from build123d import *

# Parameters (mm, degrees)
F0_R     = 1.6
F0_W     = 60
F0_H     = 15
F1_DEPTH = 2
F2_R     = 3
F3_SIZE  = 0.2


with BuildPart() as f1:
    # F0 (on Front) → F1 (new body)
    with BuildSketch(Plane.XZ):
        Polygon((-45, -57.5), (25, -57.5), (25, 0), (45, 0), (45, 57.5), (-45, 57.5), align=None)
        with Locations((-37.5, -52.5)):
            Circle(F0_R, mode=Mode.SUBTRACT)
        with Locations((-7.5, -52.5)):
            Circle(F0_R, mode=Mode.SUBTRACT)
        with Locations((-4.111738, 18.929576)):
            Rectangle(F0_W, F0_H, mode=Mode.SUBTRACT)
        with Locations((-37.5, 52.5)):
            Circle(F0_R, mode=Mode.SUBTRACT)
        with Locations((37.5, 7.5)):
            Circle(F0_R, mode=Mode.SUBTRACT)
        with Locations((37.5, 52.5)):
            Circle(F0_R, mode=Mode.SUBTRACT)
    extrude(amount=F1_DEPTH)

    # F2
    f2_edges = [f1.edges().sort_by_distance(p)[0] for p in [
        (25, -1, 0),
    ]]
    fillet(f2_edges, radius=F2_R)

    # F3
    f3_edges = [f1.edges().sort_by_distance(p)[0] for p in [
        (0, -2, 57.5),
        (0, 0, 57.5),
        (45, -1, 57.5),
        (45, 0, 28.75),
        (36.5, -2, 0),
        (45, -2, 28.75),
        (-10, -2, -57.5),
        (45, -1, 0),
        (36.5, 0, 0),
        (25, -1, -57.5),
        (-10, 0, -57.5),
        (-45, 0, 0),
        (-45, -2, 0),
        (-45, -1, 57.5),
        (-45, -1, -57.5),
    ]]
    chamfer(f3_edges, length=F3_SIZE)


solid = f1.part
Geometry: final body of the model. Coordinates: model frame, mm. Round coordinates to 2 decimals unless told otherwise and drop trailing zeros. Loops run counter-clockwise (first coordinate to the right, second up) from the corner with the lowest first, then second, coordinate; pieces in that order, holes last. Notation, with made-up numbers: M 75.5,82.5 L 88.5,82.5 A25 ccw 88.5,121.5 Z; hole C -18,38 d11. An arc over 180 degrees is marked long. Put each result on its own line as item: value. Start each with the question number.
(1) Contact query for flat-ended pins moving along their axis: pin 1 Ø0.8 at (y, z) = (-1, -28.5) entering from +X; pin 2 Ø1.9 at (x, z) = (37.5, 7.5) entering from -Y; pin 3 Ø2 at (x, z) = (-17.5, 45) entering from +Y. Output: stop coordinate, or through.
(2) Draft query along X for faces 1 (the face through (-9.1, -0.99, -52.43)), 2 (the face through (-1, 0, 1)), 3 (the face through (25.86, -1.01, -0.9)). Return one class per face: +X half, -X half, draft (parallel to the pull), parting line (faces both ways), or undercut.
(3) Section query A-A (z = -52.5). Return loops of the section in (x, y).
(4) Material intervals for line 1 along Z through (x, y) = (-37.5, -0.4); line 2 along Z through (x, y) = (-7.5, -1.45); line 3 along Z through (x, y) = (-30.5, -1.7), sorted ascending. Write a range as [from, to].
(5) Section query B-B (x = -37.5). Return loops of the section in (y, z), then the cut area to 3 significant figures.
(6) Section query D-D (x = -18.5). Return loops of the section in (y, z), then the cut area to 3 significant figures.
(7) Section query C-C (y = -0.9). Return loops of the section in (x, z).
Findings below:
1. pin 1: stops at x = 25
1. pin 2: passes through
1. pin 3: stops at y = 0
2. face 1: undercut
2. face 2: draft
2. face 3: +X half
3. outline: M -45,-1.8 L -44.8,-2 L -39.1,-2 L -39.1,0 L -44.8,0 L -45,-0.2 Z; M -35.9,-2 L -9.1,-2 L -9.1,0 L -35.9,0 Z; M -5.9,-2 L 24.8,-2 L 25,-1.8 L 25,-0.2 L 24.8,0 L -5.9,0 Z
4. line 1: z = [-57.5, -54.1], [-50.9, 50.9], [54.1, 57.5]
4. line 2: z = [-57.5, -54.1], [-50.9, 11.43], [26.43, 57.5]
4. line 3: z = [-57.5, 11.43], [26.43, 57.5]
5. outline: M -2,-57.3 L -1.8,-57.5 L -0.2,-57.5 L 0,-57.3 L 0,-54.1 L -2,-54.1 Z; M -2,-50.9 L 0,-50.9 L 0,50.9 L -2,50.9 Z; M -2,54.1 L 0,54.1 L 0,57.3 L -0.2,57.5 L -1.8,57.5 L -2,57.3 Z
5. area: 217 mm2
6. outline: M -2,-57.3 L -1.8,-57.5 L -0.2,-57.5 L 0,-57.3 L 0,11.43 L -2,11.43 Z; M -2,26.43 L 0,26.43 L 0,57.3 L -0.2,57.5 L -1.8,57.5 L -2,57.3 Z
6. area: 200 mm2
7. outline: M -45,-57.3 L -44.8,-57.5 L 24.8,-57.5 L 25,-57.3 L 25,-3 A3 cw 28,0 L 44.8,0 L 45,0.2 L 45,57.3 L 44.8,57.5 L -44.8,57.5 L -45,57.3 Z; hole C -37.5,-52.5 d3.2; hole C -37.5,52.5 d3.2; hole M -34.11,11.43 L 25.89,11.43 L 25.89,26.43 L -34.11,26.43 Z; hole C -7.5,-52.5 d3.2; hole C 37.5,7.5 d3.2; hole C 37.5,52.5 d3.2
